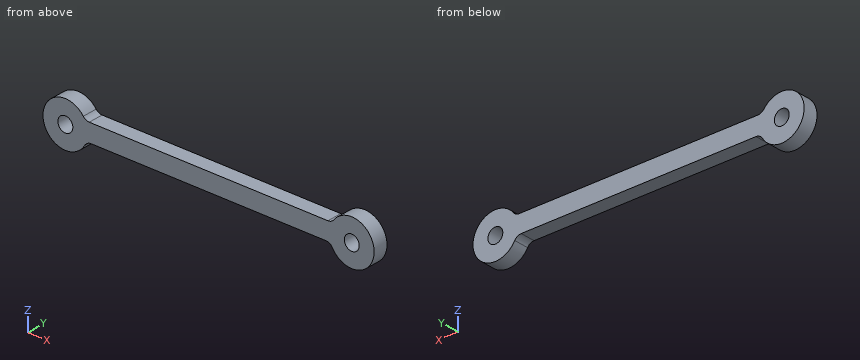
from build123d import *

# Parameters (mm, degrees)
F0_R     = 5
F1_DEPTH = 10


with BuildPart() as f1:
    # F0 (on Front) → F1 (new body)
    with BuildSketch(Plane.XZ):
        with BuildLine():
            ThreePointArc((-83.009619, -9.5), (-81.179492, -7.669873), (-78.679492, -7))
            Line((-78.679492, -7), (0, -7))
            Line((0, -7), (78.679492, -7))
            ThreePointArc((78.679492, -7), (81.179492, -7.669873), (83.009619, -9.5))
            ThreePointArc((83.009619, -9.5), (110.973052, -2.898729), (84, 7))
            ThreePointArc((84, 7), (82.236068, 5.527864), (80, 5))
            Line((80, 5), (0, 5))
            Line((0, 5), (-80, 5))
            ThreePointArc((-80, 5), (-82.236068, 5.527864), (-84, 7))
            ThreePointArc((-84, 7), (-110.973052, -2.898729), (-83.009619, -9.5))
        make_face()
        with Locations((-96, -2)):
            Circle(F0_R, mode=Mode.SUBTRACT)
        with Locations((96, -2)):
            Circle(F0_R, mode=Mode.SUBTRACT)
    extrude(amount=F1_DEPTH)


solid = f1.part
Work out the finished part from the listing and answer in its coordinate system (mm). Round coordinates to 2 decimals unless told otherwise and drop trailing zeros. Order: outer loops, then holes, each group sorted by start corner. A loop starts at its lowest first (then second) coordinate and runs counter-clockwise, first axis right, second up. Notation, with made-up numbers: M 74,18.5 L 112,18.5 A29 cw 112,41.5 Z; hole C 67,75.5 d4. An arc over 180 degrees is marked long. Put each result on its own line as item: value. Start each with the question number.
Q1. Straight lines are drawn through the part: L1, parallel to Z at x = -96, y = -4; L2, parallel to X at y = -8.25, z = -6.25; L3, parallel to X at y = -3.5, z = 0.5. For each, find the intervals that lie inside material, in ascending order. Write a range as [from, to].
Q2. Flat-ended cylindrical pins translate along their axes: pin 1 (3 mm diameter, centred on x = 37, y = -5.5, fed in from +Z); pin 2 (4 mm diameter, centred on y = -5.5, z = 4, fed in from -X); pin 3 (4 mm diameter, centred on y = -6.5, z = 8, fed in from -X). Find the tip coordinate at first contact, or state that the pin passes through.
Q3. Section A-A, the plane z = -2 is taken. Write down the section's boundary in (x, y), and give its area (3 significant figures).
Q4. Section C-C, the plane y = -5.25 is taken. Write down the section's boundary in (x, z), and give its area (3 significant figures).
Q5. Section D-D, the plane z = -12.75 is taken. Write down the section's boundary in (x, y), and give its area (3 significant figures).
Q6. Section B-B, the plane x = -96 is taken. Write down the section's boundary in (y, z).
Findings below:
1. L1: z = [-17, -7], [3, 13]
1. L2: x = [-110.39, -98.63], [-93.37, 93.37], [98.63, 110.39]
1. L3: x = [-110.79, -100.33], [-91.67, 91.67], [100.33, 110.79]
2. pin 1: stops at z = 5
2. pin 2: stops at x = -110.46
2. pin 3: stops at x = -108.69
3. outline: M -111,-10 L -101,-10 L -101,0 L -111,0 Z; M -91,-10 L 91,-10 L 91,0 L -91,0 Z; M 101,-10 L 111,-10 L 111,0 L 101,0 Z
3. area: 2,020 mm^2
4. outline: M -84,7 A15 ccw long -83.01,-9.5 A5 cw -78.68,-7 L 78.68,-7 A5 cw 83.01,-9.5 A15 ccw long 84,7 A5 cw 80,5 L -80,5 A5 cw Z; hole C -96,-2 d10; hole C 96,-2 d10
4. area: 3,220 mm^2
5. outline: M -106.46,-10 L -85.54,-10 L -85.54,0 L -106.46,0 Z; M 85.54,-10 L 106.46,-10 L 106.46,0 L 85.54,0 Z
5. area: 418 mm^2
6. outline: M -10,-17 L 0,-17 L 0,-7 L -10,-7 Z; M -10,3 L 0,3 L 0,13 L -10,13 Z
